Geometry: final body of the model. Coordinates: model frame, mm. A direction names the side the tool comes from. Give positions to 0.01 mm unless a question says otherwise; leave off trailing zeros. Loops run counter-clockwise (first coordinate to the right, second up) from the corner with the lowest first, then second, coordinate; pieces in that order, holes last. Notation, with made-up numbers: (-23, 44.5) - (-12, 44.5) arc R15 cw to (-12, 61.5) - close; hole circle Ø8 at (-35, -36.5). An arc over 180 degrees is marked (long way). Answer in a Markdown table with one row per item.
Autodesk Inventor part; units mm, degrees
ref_plane "YZ Plane" through (0, 0, 0) normal (1, 0, 0) x (0, 1, 0)
ref_plane "XZ Plane" through (0, 0, 0) normal (0, 1, 0) x (-1, 0, 0)
ref_plane "XY Plane" through (0, 0, 0) normal (0, 0, 1) x (1, 0, 0)
sketch "Sketch1" plane through (0, 0, 0) normal (0, 1, 0) x (-1, 0, 0)
  line L0 (0, 0) -> (0, -197.866) construction
  line L1 (-6.35, 0) -> (-6.35, -197.866)
  line L2 (6.35, -197.866) -> (6.35, 0)
  arc A0 (6.35, 0) -> (-6.35, 0) centre (0, 0) ccw
  arc A1 (-6.35, -197.866) -> (6.35, -197.866) centre (0, -197.866) ccw
  circle A2 centre (0, 0) radius 2.2987
  line L3 (0, -98.933) -> (6.35, -98.933)
  circle A3 centre (0, -197.866) radius 2.2987
  line L4 (-6.35, 6.35) -> (6.35, 6.35)
  line L5 (6.35, 6.35) -> (6.35, -6.35)
  line L6 (6.35, -6.35) -> (-6.35, -6.35)
  line L7 (-6.35, -6.35) -> (-6.35, 6.35)
  line L8 (-6.35, 6.35) -> (6.35, -6.35) construction
  line L9 (6.35, 6.35) -> (-6.35, -6.35) construction
  line L10 (-6.35, -204.216) -> (6.35, -204.216)
  line L11 (6.35, -204.216) -> (6.35, -191.516)
  line L12 (6.35, -191.516) -> (-6.35, -191.516)
  line L13 (-6.35, -191.516) -> (-6.35, -204.216)
  line L14 (-6.35, -204.216) -> (6.35, -191.516) construction
  line L15 (6.35, -204.216) -> (-6.35, -191.516) construction
  dimension "d0" = 197.866
  dimension "d1" = 12.7
  dimension "d2" = 4.5974
  dimension "d3" = 12.7
  dimension "d4" = 12.7
  dimension "d5" = 12.7
  dimension "d6" = 12.7
extrude "Extrusion1" add sketch "Sketch1" along normal blind 12.7 contours L6 L2 L12 L1
extrude "Extrusion2" add sketch "Sketch1" along normal blind 6.35 contours A0 L2 L6 L1 | L12 L2 A1 L1
chamfer "Chamfer1" distance 3.175 angle 45 2 edges at (2.2987, 6.35, 0) (2.2987, 6.35, -197.866)
sketch "Sketch2" plane through (6.35, 12.7, -6.35) normal (1, 0, 0) x (0, 0, -1)
  line L0 (-6.35, -12.7) -> (191.516, -12.7)
  line L1 (191.516, -12.7) -> (191.516, -6.35)
  line L2 (185.166, -6.35) -> (191.516, -6.35)
  line L3 (185.166, -6.35) -> (185.166, 0)
  line L4 (0, 0) -> (185.166, 0)
  line L5 (0, -6.35) -> (0, 0)
  line L6 (-6.35, -6.35) -> (0, -6.35)
  line L7 (-6.35, -12.7) -> (-6.35, -6.35)
  line L8 (0, -6.35) -> (0, -12.7)
  line L9 (185.166, -6.35) -> (185.166, -12.7)
  line L10 (0, -6.35) -> (6.3485, -6.35)
  line L11 (185.166, -6.35) -> (178.816, -6.35)
  circle A0 centre (6.3485, -6.35) radius 4.8895
  line L12 (178.816, -6.35) -> (21.4671, -6.35) construction
  line L13 (178.816, -1.4605) -> (21.4671, -1.4605)
  line L14 (21.4671, -11.2395) -> (178.816, -11.2395)
  arc A1 (178.816, -11.2395) -> (178.816, -1.4605) centre (178.816, -6.35) ccw
  arc A2 (21.4671, -1.4605) -> (21.4671, -11.2395) centre (21.4671, -6.35) ccw
  point P0 (100.1415, -6.35)
  dimension "d14" = 6.35
  dimension "d15" = 9.779
  dimension "d16" = 9.779
extrude "Extrusion3" cut sketch "Sketch2" against normal blind 33.3375 contours A1 L14 A2 L13 | A0
sketch "Sketch3" plane through (6.35, 0, 0) normal (1, 0, 0) x (0, 0, -1)
  circle A0 centre (12.6985, 6.35) radius 4.8895
  arc A1 (27.8171, 11.2395) -> (27.8171, 1.4605) centre (27.8171, 6.35) ccw
  line L0 (27.8171, 11.2395) -> (185.166, 11.2395)
  arc A2 (185.166, 1.4605) -> (185.166, 11.2395) centre (185.166, 6.35) ccw
  line L1 (185.166, 1.4605) -> (27.8171, 1.4605)
  arc A3 (27.8171, 11.2395) -> (27.8171, 1.4605) centre (27.8171, 6.35) ccw
  circle A4 centre (12.6985, 6.35) radius 4.8895
  line L2 (6.35, 6.35) -> (6.35, 12.7)
  line L3 (0, 6.35) -> (6.35, 6.35)
  line L4 (0, 0) -> (0, 6.35)
  line L5 (0, 0) -> (197.866, 0)
  line L6 (197.866, 0) -> (197.866, 6.35)
  line L7 (191.516, 6.35) -> (197.866, 6.35)
  line L8 (191.516, 6.35) -> (191.516, 12.7)
  line L9 (6.35, 12.7) -> (191.516, 12.7)
  line L10 (12.6985, 6.35) -> (134.6504, 128.3019) construction
  line L11 (17.1887, 1.8599) -> (139.1405, 123.8118)
  line L12 (130.1603, 132.792) -> (8.2084, 10.8401)
  arc A5 (8.2084, 10.8401) -> (17.1887, 1.8599) centre (12.6985, 6.35) ccw
  arc A6 (139.1405, 123.8118) -> (130.1603, 132.792) centre (134.6504, 128.3019) ccw
  line L13 (12.6985, 6.35) -> (185.1645, 6.35) construction
  line L14 (73.6745, 67.3259) -> (134.6504, 6.35)
  line L15 (134.6504, 6.35) -> (12.6985, 128.3019) construction
  line L16 (139.1405, 10.8401) -> (17.1887, 132.792)
  line L17 (8.2084, 123.8118) -> (130.1603, 1.8599)
  arc A7 (130.1603, 1.8599) -> (139.1405, 10.8401) centre (134.6504, 6.35) ccw
  arc A8 (17.1887, 132.792) -> (8.2084, 123.8118) centre (12.6985, 128.3019) ccw
  circle A9 centre (73.6745, 67.3259) radius 4.8895
  dimension "d20" = 172.466
  dimension "d21" = 45
  dimension "d22" = 12.7
  dimension "d23" = 172.466
  dimension "d24" = 12.7
  dimension "d25" = 9.779
  dimension "d26" = 9.779
extrude "Extrusion4" add sketch "Sketch1" against normal blind 1.5875 contours A0 L2 L6 L1 | L6 L2 L12 L1 | L12 L2 A1 L1
sketch "Sketch4" plane through (0, 12.7, 0) normal (0, 1, 0) x (1, 0, 0)
  line L0 (6.35, 6.35) -> (6.35, 191.516)
  line L1 (-6.35, 191.516) -> (-6.35, 6.35)
  line L2 (-6.35, 6.35) -> (6.35, 6.35)
  line L3 (6.35, 191.516) -> (-6.35, 191.516)
  point P0 (0, 0)
extrude "Extrusion5" add sketch "Sketch4" along normal blind 1.5875
fillet "Fillet2" radius 1.27 4 edges at (0, 14.2875, -191.516) (0, 6.35, -191.516) (0, 6.35, -6.35) (0, 14.2875, -6.35)
properties part number "Scissor Base"
Q1. Cut plane B-B (x = 0). Give the number of separate pieces and of enclosed holes in the cut face, and give its area (3 significant figures).
Check values:
| item | result |
|---|---|
| separate pieces | 3 |
| enclosed holes | 2 |
| area | 1,360 mm² |
Q2. Material intervals for line 1 along Y through (x, z) = (-1.25, -146.5); line 2 along Z through (x, y) = (0, 1); line 3 along Z through (x, y) = (0, 2.15), sorted ascending.
Check values:
| item | result |
|---|---|
| line 1 | -1.59 to 1.46, 11.24 to 14.29 |
| line 2 | -204.22 to -200.16, -195.57 to -2.3, 2.3 to 6.35 |
| line 3 | -204.22 to -200.16, -195.57 to -187.67, -25.31 to -15.2, -10.2 to -2.3, 2.3 to 6.35 |
Q3. Cut plane A-A (z = -36). Output: boundary loops of the cut face in (x, y).
Check values:
| item | result |
|---|---|
| outline | (-6.35, -1.59) - (6.35, -1.59) - (6.35, 1.46) - (-6.35, 1.46) - close; (-6.35, 11.24) - (6.35, 11.24) - (6.35, 14.29) - (-6.35, 14.29) - close |
Q4. Draft query along Y for faces 6 (the conical face through (0.541, 3.374, -2.438)), 7 (the flat face through (0, -1.588, -97)), 8 (the flat face through (0, 11.24, -108)), 9 (the cylindrical face through (0.299, 0.827, -195.587)). Return one class per face: pulls with the +Y half, pulls with the -Y half, needs draft (parallel to the pull), parting line crosses it, or undercut.
Check values:
| item | result |
|---|---|
| face 6 | pulls with the +Y half |
| face 7 | pulls with the -Y half |
| face 8 | undercut |
| face 9 | needs draft |
Q5. First-contact query: pin 1 (3 mm diameter, centred on x = 0, z = -197.866, fed in from +Y) (3 decimals); pin 2 (6 mm diameter, centred on x = -2, y = 10, fed in from +Z); pin 3 (1.5 mm diameter, centred on x = -4.5, y = 2.5, fed in from +Z); pin 4 (4.5 mm diameter, centred on x = 1, y = 11.5, fed in from -Z). Flat tips, straight axial feed; report the tip coordinate or a pass-through.
Check values:
| item | result |
|---|---|
| pin 1 | through |
| pin 2 | z = -6.19 |
| pin 3 | z = 5.12 |
| pin 4 | z = -191.52 |
Q6. Reachability of faces 1 (the flat face through (0, 10, -6.35)), 2 (the conical face through (0.54, 3.37, -200.3)), 3 (the cylindrical face through (0.14, 2.33, 6.35)), 4 (the flat face through (0, 10, -191.516)), 5 (the cylindrical face through (0.09, 6.46, -22.93)) from +Z, -Z, +X, -X, +Y, -Y: full face, straight path, thin tool, end or side. Return the list, or none.
Check values:
| item | result |
|---|---|
| face 1 | +Z, +X, -X, +Y |
| face 2 | +Y |
| face 3 | +Z, +Y, -Y |
| face 4 | -Z, +X, -X, +Y |
| face 5 | +X, -X |
